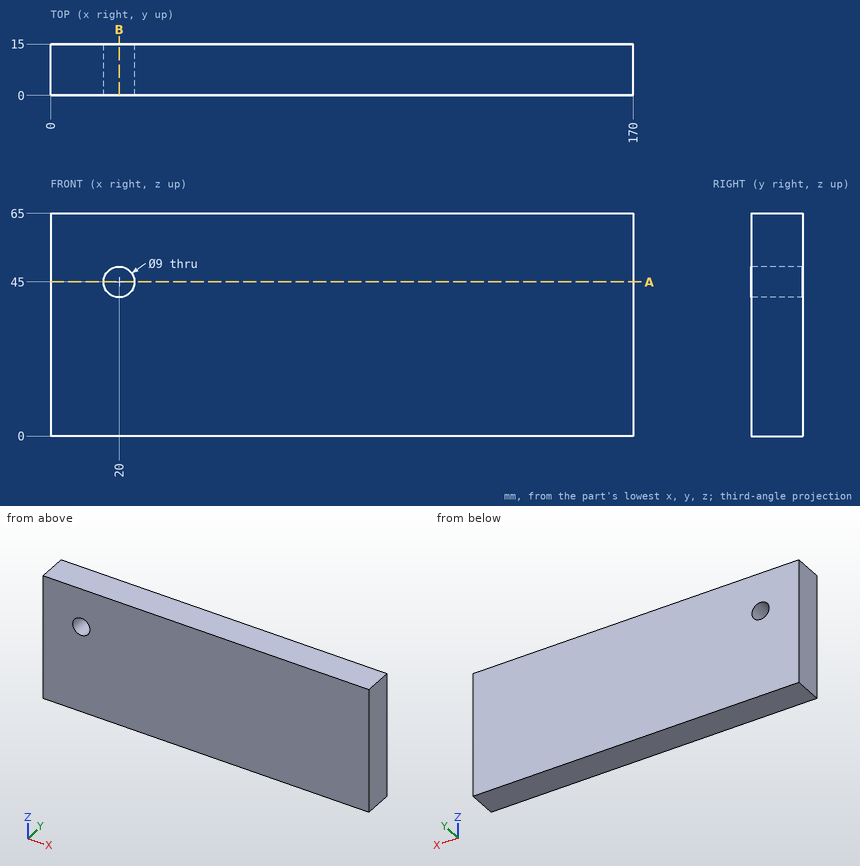
Source: three-view drawing plus pictorial views. Frame: mm from the lowest corner of the part. Give positions to 0.01 mm unless a question says otherwise; leave off trailing zeros. Order: outer loops, then holes, each group sorted by start corner. A loop starts at its lowest first (then second) coordinate and runs counter-clockwise, first axis right, second up. Notation, with made-up numbers: M 81,22.25 L 85,22.25 A29 ccw 85,60.25 Z; hole C 72.5,38.25 d5. An arc over 180 degrees is marked long. One line per question, with ' | ' between items. Start each with the question number.
1. Section query B-B (x = 20). Return the cut outline in (y, z).
2. Material intervals for probe 1 along Z at (x, y) = (20, 12); probe 2 along X at (y, z) = (12.75, 47); probe 3 along X at (y, z) = (4, 43.5), sorted ascending. Write a range as [from, to].
3. Section query A-A (z = 45). Return the cut outline in (x, y).
Here are the results:
1) outline: M 0,0 L 15,0 L 15,40.5 L 0,40.5 Z; M 0,49.5 L 15,49.5 L 15,65 L 0,65 Z
2) probe 1: [0, 40.5], [49.5, 65] | probe 2: [0, 15.97], [24.03, 170] | probe 3: [0, 15.76], [24.24, 170]
3) outline: M 0,0 L 15.5,0 L 15.5,15 L 0,15 Z; M 24.5,0 L 170,0 L 170,15 L 24.5,15 Z
